```python
from build123d import *

# Parameters (mm, degrees)
SKETCH1_R           = 45
BOSS_EXTRUDE1_DEPTH = 80
SKETCH2_R           = 45
SKETCH2_R_2         = 40
CUT_EXTRUDE3_DEPTH  = 10
SKETCH3_R           = 32.5
CUT_EXTRUDE4_DEPTH  = 103.225241501


with BuildPart() as part:
    # Sketch1 → Boss-Extrude1 (new body)
    with BuildSketch(Plane(origin=(0, 0, 0), x_dir=(1, 0, 0), z_dir=(0, 1, 0))):
        with Locations(Location((0, 0, 0), (0, 0, 270))):
            Circle(SKETCH1_R)
    extrude(amount=BOSS_EXTRUDE1_DEPTH)

    # Sketch2 → Cut-Extrude3 (cut)
    with BuildSketch(Plane.XZ):
        with Locations(Location((0, 0, 0), (0, 0, 270))):
            Circle(SKETCH2_R)
        with Locations(Location((0, 0, 0), (0, 0, 270))):
            Circle(SKETCH2_R_2, mode=Mode.SUBTRACT)
    extrude(amount=-CUT_EXTRUDE3_DEPTH, mode=Mode.SUBTRACT)

    # Sketch3 → Cut-Extrude4 (cut, through all)
    with BuildSketch(Plane.XZ):
        with Locations(Location((0, 0, 0), (0, 0, 270))):
            Circle(SKETCH3_R)
    extrude(amount=-CUT_EXTRUDE4_DEPTH, mode=Mode.SUBTRACT)


solid = part.part
```
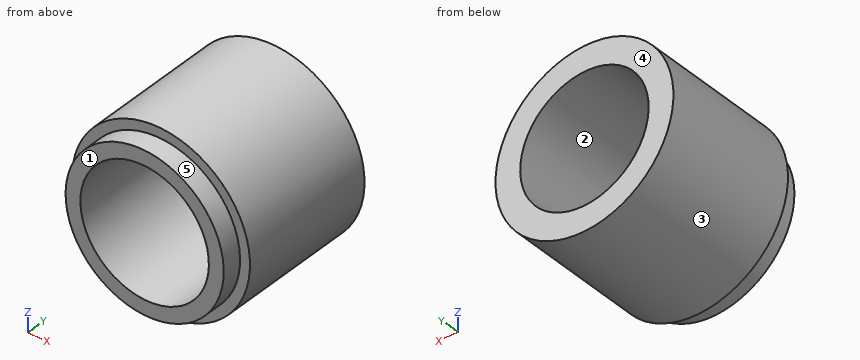
Part model, mm, in its own coordinate system. Face numbers are marked on the shaded views. A direction names the side the tool comes from. Round coordinates to 2 decimals unless told otherwise and drop trailing zeros. Loops run counter-clockwise (first coordinate to the right, second up) from the corner with the lowest first, then second, coordinate; pieces in that order, holes last.
1. Drill centre lines: line 1 along X through (y, z) = (37, 0); line 2 along X through (y, z) = (17, 13). Where is each one in solid material? Low to high.
Solutions:
line 1: x = -45 to -32.5, 32.5 to 45
line 2: x = -43.08 to -29.79, 29.79 to 43.08
2. Slice it at C-C (y = 43). Give the cut face in (x, z).
Solutions:
outline: circle Ø90 at (0, 0); hole circle Ø65 at (0, 0)
3. Flat gauge pins, fed straight in: pin 1 (3 mm diameter, centred on y = 22, z = 28, fed in from -X); pin 2 (1 mm diameter, centred on x = 2.5, y = 19, fed in from -Z); pin 3 (6 mm diameter, centred on y = 40.5, z = 2.5, fed in from -X). Where does each tip first touch, or does it go through?
Solutions:
pin 1: stops at x = -36.37
pin 2: stops at z = -44.96
pin 3: stops at x = -45
4. Slice it at A-A (z = 0). Give the cut face in (x, y), and give its area (3 significant figures).
Solutions:
outline: (-45, 10) - (-40, 10) - (-40, 0) - (-32.5, 0) - (-32.5, 80) - (-45, 80) - close; (32.5, 0) - (40, 0) - (40, 10) - (45, 10) - (45, 80) - (32.5, 80) - close
area: 1,900 mm2
5. Two-plate mould, pull along X, no slides. Class the marked faces 1, 2 and 3: pulls with the +X half, pulls with the -X half, needs draft (parallel to the pull), parting line crosses it, or undercut.
Solutions:
face 1: needs draft
face 2: undercut
face 3: parting line crosses it
6. 3-axis set-ups, long thin cutter, end or side, ignore diameter. For the marked faces 4 and 5: which of +Z, -Z, +X, -X, +Y, -Y reach the whole face in a straight line?
Solutions:
face 4: +Z, -Z, +X, -X, +Y
face 5: -Y
7. Slice it at D-D (x = -34.5). Give the cut face in (y, z).
Solutions:
outline: (0, -20.24) - (10, -20.24) - (10, -28.89) - (80, -28.89) - (80, 28.89) - (10, 28.89) - (10, 20.24) - (0, 20.24) - close
8. Slice it at B-B (x = 0). Give the cut face in (y, z).
Solutions:
outline: (0, -40) - (10, -40) - (10, -45) - (80, -45) - (80, -32.5) - (0, -32.5) - close; (0, 32.5) - (80, 32.5) - (80, 45) - (10, 45) - (10, 40) - (0, 40) - close
